Here's how the part is built. I have some questions about the finished solid (model axes, mm). A direction names the side the tool comes from. Round coordinates to 2 decimals unless told otherwise and drop trailing zeros. Write each loop counter-clockwise with the first axis right and the second up, starting at its lowest first coordinate (ties: lowest second). Pieces come first, ordered by that corner, then holes. Notation, with made-up numbers: (41, -10) - (77, -10) arc R18 ccw to (77, 12) - close; hole circle Ø9 at (23, 76.5). An arc over 180 degrees is marked (long way). Use one line per item in the form item = value. Start each with the question number.
1. I want a section at A-A, the plane z = -14. List the corners of the cut face in (x, y) for me.
2. I want a section at D-D, the plane z = 1.5. List the corners of the cut face in (x, y) for me.
3. I want a section at C-C, the plane y = -9. List the corners of the cut face in (x, z) for me, plus the area to 4 significant figures.
4. I want a section at B-B, the plane x = 16. List the corners of the cut face in (y, z) for me.
5. We'd pull the mould along Z, two halves only. Please class faces 5 (the cylindrical face through (18.146, 20.014, -14.676)), 6 (the flat face through (50, 20, 0)), 7 (the flat face through (2, 0, -24.5)): +Z half, -Z half, draft (parallel to the pull), parting line (faces both ways), or undercut.
6. If I drill on line 1 along Z through (x, y) = (16, 20); line 2 along X through (y, z) = (20.25, -14); line 3 along X through (y, z) = (-9, 7), over which ranges is the centre line in solid material (lowest first)?
7. Will these pins go through, and if not, where does the flat tip stop? pin 1 (24.5 mm diameter, centred on y = -3.5, z = -11.5, fed in from +X); pin 2 (21 mm diameter, centred on x = 31.5, z = -0.5, fed in from +Y); pin 3 (21 mm diameter, centred on x = 31, y = 3, fed in from +Z); pin 4 (4 mm diameter, centred on x = 16, z = -14, fed in from +Y).
8. Which directions (+Z, -Z, +X, -X, +Y, -Y) give clear straight access to the entire face, cutting with the end or side of a thin tool? Please do faces 1 (the flat face through (19, 0, 7)), 2 (the flat face through (21, 0, 0)), 3 (the flat face through (19, 0, -7)), 4 (the flat face through (9, 3, -21)).
```python
from build123d import *

# Parameters (mm, degrees)
SKETCH1_W                  = 49
SKETCH1_H                  = 49
BOSS_EXTRUDE1_DEPTH        = 4.5
SKETCH3_W                  = 42
SKETCH3_H                  = 42
BOSS_EXTRUDE3_DEPTH        = 5.5
SKETCH4_W                  = 42
SKETCH4_H                  = 2
BOSS_EXTRUDE4_DEPTH        = 40
SKETCH5_W                  = 10
SKETCH5_H                  = 38
BOSS_EXTRUDE5_DEPTH        = 11
SKETCH6_W                  = 2
SKETCH6_H                  = 38
BOSS_EXTRUDE6_DEPTH        = 3.5
SKETCH7_W                  = 2
SKETCH7_H                  = 38
BOSS_EXTRUDE7_DEPTH        = 3.5
F_4_5_4_5_DIAMETER_SLOT1_D = 4.5


with BuildPart() as part:
    # Sketch1 → Boss-Extrude1 (new body)
    with BuildSketch(Plane(origin=(0, 0, 0), x_dir=(0, 0, -1), z_dir=(1, 0, 0))):
        Rectangle(SKETCH1_W, SKETCH1_H)
    extrude(amount=BOSS_EXTRUDE1_DEPTH)

    # Sketch3 → Boss-Extrude3 (add)
    with BuildSketch(Plane(origin=(4.5, 0, 0), x_dir=(0, 0, -1), z_dir=(1, 0, 0))):
        Rectangle(SKETCH3_W, SKETCH3_H)
    extrude(amount=BOSS_EXTRUDE3_DEPTH)

    # Sketch4 → Boss-Extrude4 (add)
    with BuildSketch(Plane(origin=(10, 0, 0), x_dir=(0, 0, -1), z_dir=(1, 0, 0))):
        with Locations((0, 20)):
            Rectangle(SKETCH4_W, SKETCH4_H)
    extrude(amount=BOSS_EXTRUDE4_DEPTH)

    # Sketch5 → Boss-Extrude5 (add)
    with BuildSketch(Plane(origin=(10, 0, 0), x_dir=(0, 0, -1), z_dir=(1, 0, 0))):
        Rectangle(SKETCH5_W, SKETCH5_H)
    extrude(amount=BOSS_EXTRUDE5_DEPTH)

    # Sketch6 → Boss-Extrude6 (add)
    with BuildSketch(Plane.XY.offset(5)):
        with Locations((18, 0)):
            Rectangle(SKETCH6_W, SKETCH6_H)
    extrude(amount=BOSS_EXTRUDE6_DEPTH)

    # Sketch7 → Boss-Extrude7 (add)
    with BuildSketch(Plane(origin=(0, 0, -5), x_dir=(-1, 0, 0), z_dir=(0, 0, -1))):
        with Locations((-18, 0)):
            Rectangle(SKETCH7_W, SKETCH7_H)
    extrude(amount=BOSS_EXTRUDE7_DEPTH)

    # Ø4.5 (4.5) Diameter Slot1 (through all)
    with Locations(Plane(origin=(0, 19, 0), x_dir=(-1, 0, 0), z_dir=(0, -1, 0))):
        with Locations((-44, 14), (-44, -14), (-16, -14), (-16, 14)):
            Hole(F_4_5_4_5_DIAMETER_SLOT1_D / 2)


solid = part.part
```
Model answer:
q1.outline = (0, -24.5) - (4.5, -24.5) - (4.5, -21) - (10, -21) - (10, 19) - (13.75, 19) - (13.75, 21) - (4.5, 21) - (4.5, 24.5) - (0, 24.5) - close; (18.25, 19) - (41.75, 19) - (41.75, 21) - (18.25, 21) - close; (46.25, 19) - (50, 19) - (50, 21) - (46.25, 21) - close
q2.outline = (0, -24.5) - (4.5, -24.5) - (4.5, -21) - (10, -21) - (10, -19) - (21, -19) - (21, 19) - (50, 19) - (50, 21) - (4.5, 21) - (4.5, 24.5) - (0, 24.5) - close
q3.outline = (0, -24.5) - (4.5, -24.5) - (4.5, -21) - (10, -21) - (10, -5) - (17, -5) - (17, -8.5) - (19, -8.5) - (19, -5) - (21, -5) - (21, 5) - (19, 5) - (19, 8.5) - (17, 8.5) - (17, 5) - (10, 5) - (10, 21) - (4.5, 21) - (4.5, 24.5) - (0, 24.5) - close
q3.area = 575.5 mm2
q4.outline = (-19, -5) - (19, -5) - (19, -11.75) - (21, -11.75) - (21, 11.75) - (19, 11.75) - (19, 5) - (-19, 5) - close; (19, -21) - (21, -21) - (21, -16.25) - (19, -16.25) - close; (19, 16.25) - (21, 16.25) - (21, 21) - (19, 21) - close
q5.face_5 = undercut
q5.face_6 = draft
q5.face_7 = -Z half
q6.line_1 = -21 to -16.25, -11.75 to 11.75, 16.25 to 21
q6.line_2 = 0 to 13.75, 18.25 to 41.75, 46.25 to 50
q6.line_3 = 0 to 10, 17 to 19
q7.pin_1 = 21
q7.pin_2 = 21
q7.pin_3 = 5
q7.pin_4 = through
q8.face_1 = +Z, +X, -Y
q8.face_2 = +Z, -Z, +X, -Y
q8.face_3 = -Z, +X, -Y
q8.face_4 = -Z, +X, +Y, -Y
